from build123d import *

# Parameters (mm, degrees)
SKETCH_1_W      = 155
SKETCH_1_H      = 55
EXTRUDE_1_DEPTH = 1.5
FILLET_1_R      = 3.5
SKETCH_2_W      = 150
SKETCH_2_H      = 50
EXTRUDE_2_DEPTH = 1
FILLET_3_R      = 2


with BuildPart() as part:
    # 草图1 → 凸台-拉伸1 (new body)
    with BuildSketch(Plane.XY):
        with Locations((77.5, -27.5)):
            Rectangle(SKETCH_1_W, SKETCH_1_H)
    extrude(amount=EXTRUDE_1_DEPTH)

    # 圆角1
    fillet_1_edges = [part.edges().sort_by_distance(p)[0] for p in [
        (0, 0, 0.75),
        (155, 0, 0.75),
        (155, -55, 0.75),
        (0, -55, 0.75),
    ]]
    fillet(fillet_1_edges, radius=FILLET_1_R)

    # 草图2 → 凸台-拉伸2 (add)
    with BuildSketch(Plane.XY.offset(1.5)):
        with Locations((77.5, -27.5)):
            Rectangle(SKETCH_2_W, SKETCH_2_H)
    extrude(amount=EXTRUDE_2_DEPTH)

    # 圆角3
    fillet_3_edges = [part.edges().sort_by_distance(p)[0] for p in [
        (2.5, -2.5, 2),
        (2.5, -52.5, 2),
        (152.5, -52.5, 2),
        (152.5, -2.5, 2),
    ]]
    fillet(fillet_3_edges, radius=FILLET_3_R)


solid = part.part
Verification items for the finished model (mm, model axes). Coordinates: 2 decimals unless noted, no trailing zeros. Write each loop counter-clockwise with the first axis right and the second up, starting at its lowest first coordinate (ties: lowest second). Pieces come first, ordered by that corner, then holes. Notation, with made-up numbers: (89.25, 65) -> (100.25, 65) arc R22 ccw to (100.25, 73) -> close; hole circle Ø7 at (68.25, 8). An arc over 180 degrees is marked (long way). One line per item, written item: value. Start each with the question number.
Q1. Cross-section at A-A on x = 108. Enter the section's corners in (y, z).
Q2. Thickness scan on L1, parallel to X at y = -44, z = 1.55; L2, parallel to Y at x = 7, z = 1.6. Record the ranges inside material, lowest first. Write a range as from..to.
Q3. Go/stop test with flat-tipped pins: P1, Ø0.8, axis at y = -21, z = 2, coming from the -X side; P2, Ø0.8, axis at y = -34.5, z = 2, coming from the +X side; P3, Ø0.5, axis at x = 90.5, z = 2, coming from the +Y side. Record where each tip stops, or that it passes through.
Checked values:
1. outline: (-55, 0) -> (0, 0) -> (0, 1.5) -> (-2.5, 1.5) -> (-2.5, 2.5) -> (-52.5, 2.5) -> (-52.5, 1.5) -> (-55, 1.5) -> close
2. L1: x = 2.5..152.5
2. L2: y = -52.5..-2.5
3. P1: stops at x = 2.5
3. P2: stops at x = 152.5
3. P3: stops at y = -2.5
